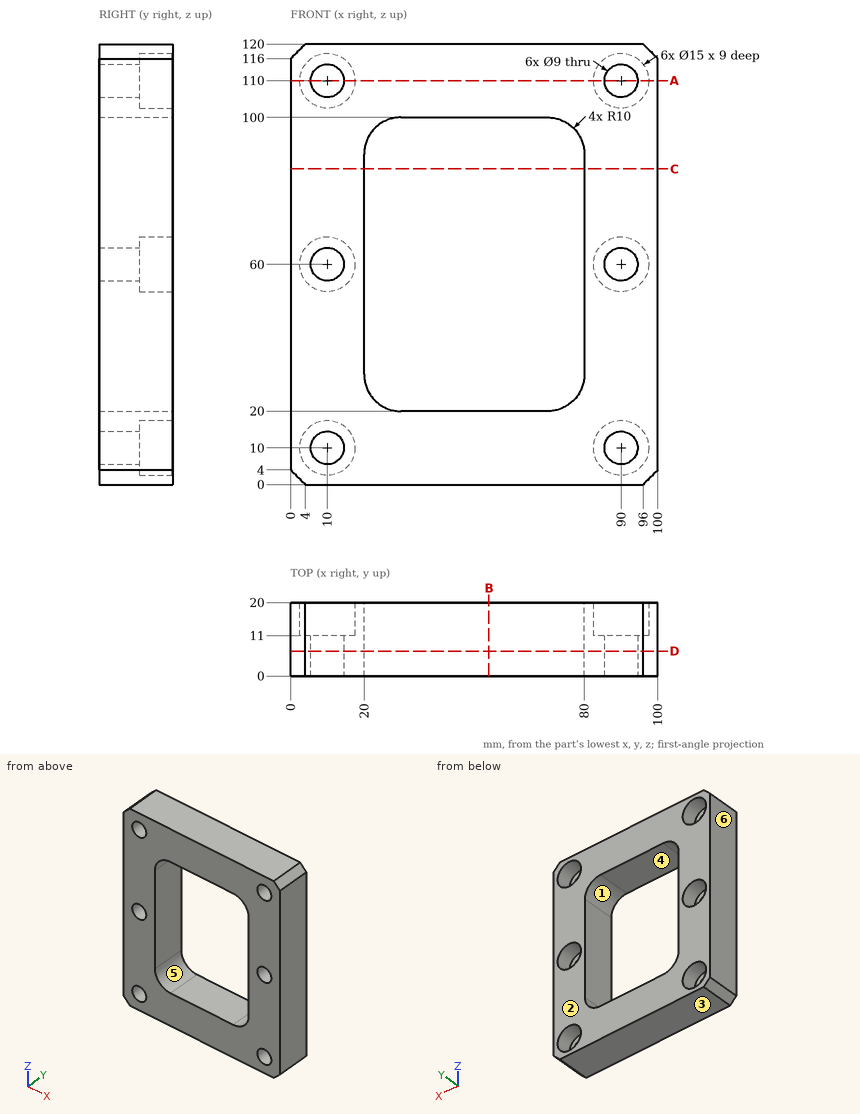
For this review, use the dimensioned drawing (mm, ordinates from the lowest corner) and the shaded views. A direction names the side the tool comes from. Coordinates: 2 decimals unless noted, no trailing zeros. Loops run counter-clockwise (first coordinate to the right, second up) from the corner with the lowest first, then second, coordinate; pieces in that order, holes last. Notation, with made-up numbers: (32.5, -21) - (66.5, -21) arc R17 ccw to (66.5, -3) - close; hole circle Ø10 at (53.5, 79.25). An arc over 180 degrees is marked (long way). Use one line per item in the form item = value. Start each with the question number.
1) For the marked faces 1 and 2, list the 3-axis set-ups (+Z, -Z, +X, -X, +Y, -Y) from which the entire face can be reached by the end or side of a thin tool; tool diameter is ignored.
2) Take a section at C-C (z = 86). State the section outline as (x, y) points, plus the area to 3 significant figures.
3) Take a section at D-D (y = 6.75). State the section outline as (x, z) points.
4) For pin 1 (7.5 mm diameter, centred on x = 8.5, z = 113, fed in from +Y); pin 2 (6 mm diameter, centred on y = 12, z = 55, fed in from -X), all flat-tipped, find the tip position at first contact; note any pin that passes through.
5) Draft analysis for pull direction Z (two halves, no side actions). For the marked faces 3, 4, 5 and 6, state which applies: released by +Z, released by -Z, zero draft, split by the parting line, or undercut.
6) Take a section at B-B (x = 54). State the section outline as (y, z) points, plus the area to 3 significant figures.
7) Take a section at A-A (z = 110). State the section outline as (x, y) points.
8) To check wall thickness, follow probe 1 along X at (y, z) = (15, 110); probe 2 along X at (y, z) = (5, 110); probe 3 along Z at (x, y) = (10, 15.25). State the ranges of each line that lie inside material, in increasing order. Write a range as from..to.
From the geometry:
q1.face_1 = +Y, -Y
q1.face_2 = +Z, -Z, +X, -X, +Y
q2.outline = (0, 0) - (20, 0) - (20, 20) - (0, 20) - close; (80, 0) - (100, 0) - (100, 20) - (80, 20) - close
q2.area = 800 mm2
q3.outline = (0, 4) - (4, 0) - (96, 0) - (100, 4) - (100, 116) - (96, 120) - (4, 120) - (0, 116) - close; hole circle Ø9 at (10, 10); hole circle Ø9 at (10, 60); hole circle Ø9 at (10, 110); hole (20, 30) arc R10 ccw to (30, 20) - (70, 20) arc R10 ccw to (80, 30) - (80, 90) arc R10 ccw to (70, 100) - (30, 100) arc R10 ccw to (20, 90) - close; hole circle Ø9 at (90, 10); hole circle Ø9 at (90, 60); hole circle Ø9 at (90, 110)
q4.pin_1 = 11
q4.pin_2 = 0
q5.face_3 = released by -Z
q5.face_4 = undercut
q5.face_5 = undercut
q5.face_6 = zero draft
q6.outline = (0, 0) - (20, 0) - (20, 20) - (0, 20) - close; (0, 100) - (20, 100) - (20, 120) - (0, 120) - close
q6.area = 800 mm2
q7.outline = (0, 0) - (5.5, 0) - (5.5, 11) - (2.5, 11) - (2.5, 20) - (0, 20) - close; (14.5, 0) - (85.5, 0) - (85.5, 11) - (82.5, 11) - (82.5, 20) - (17.5, 20) - (17.5, 11) - (14.5, 11) - close; (94.5, 0) - (100, 0) - (100, 20) - (97.5, 20) - (97.5, 11) - (94.5, 11) - close
q8.probe_1 = 0..2.5, 17.5..82.5, 97.5..100
q8.probe_2 = 0..5.5, 14.5..85.5, 94.5..100
q8.probe_3 = 0..2.5, 17.5..52.5, 67.5..102.5, 117.5..120
